For this review, take the finished solid that the model builds, in its own axes (mm). A direction names the side the tool comes from. Coordinates: 2 decimals unless noted, no trailing zeros. Write each loop counter-clockwise with the first axis right and the second up, starting at its lowest first coordinate (ties: lowest second). Pieces come first, ordered by that corner, then holes. Notation, with made-up numbers: (87, -39.5) - (114, -39.5) arc R38 cw to (114, -1.5) - close; hole circle Ø10 at (-25, 5). An arc over 180 degrees is marked (long way). Use one line per item in the form item = value. Start each with the question number.
1) For L1, parallel to Y at x = 0, z = -1; L2, parallel to Z at x = -1, y = -18.5; L3, parallel to Z at x = -15, y = 5.5, list the stretches that pass through material, from the lowest coordinate up. Write a range as from..to.
2) Tool access review of faces 5 (the flat face through (-17, 0, -52)), 6 (the cylindrical face through (-3.22, 24.54, -30.57)), 7 (the flat face through (0, -17, -5)): name each direction out of +Z, -Z, +X, -X, +Y, -Y from which nothing blocks a thin tool from reaching the whole face with its end or side.
3) We need section D-D (x = 17.5). Give the boundary of the cut face in (y, z), plus the area to 3 significant figures.
4) Insertion check: P1, Ø5, axis at x = 17.5, y = 0, coming from the -Z side; P2, Ø5, axis at y = 17.5, z = -47, coming from the -X side; P3, Ø4.5, axis at x = -17.5, y = 0, coming from the +Z side; P4, Ø10, axis at x = 5, y = 4, coming from the +Z side. Each pin has a flat end and moves straight along its axis. Give the tip position at first contact, or say it passes through.
5) We need section B-B (z = -58.5). Give the boundary of the cut face in (x, y), plus the area to 3 significant figures.
6) Mouldability with a two-part tool opening along X and no side actions: class faces 1 (the flat face through (0, 18, -5)), 2 (the cylindrical face through (1.172, 8.923, -65.451)), 3 (the flat face through (11, 0, -62)), 4 (the cylindrical face through (15.9, -1.2, -2.5)) as pulls with the +X half, pulls with the -X half, needs draft (parallel to the pull), parting line crosses it, or undercut.
7) We need section C-C (y = 17.5). Give the boundary of the cut face in (x, z), plus the area to 3 significant figures.
```python
from build123d import *

# Parameters (mm, degrees)
SKETCH1_R               = 24.75
BOSS_EXTRUDE1_DEPTH     = 62
SKETCH2_R               = 3
BOSS_EXTRUDE2_DEPTH     = 44
SKETCH3_R               = 1.1
CUT_EXTRUDE1_DEPTH      = 25.75
CUT_EXTRUDE1_DEPTH_BACK = 25.75
SKETCH4_R               = 9
BOSS_EXTRUDE3_DEPTH     = 7
SKETCH5_R               = 2
CUT_EXTRUDE2_DEPTH      = 10
SKETCH6_R               = 2
CUT_EXTRUDE3_DEPTH      = 5


with BuildPart() as part:
    # Sketch1 → Boss-Extrude1 (new body)
    with BuildSketch(Plane.XY):
        Circle(SKETCH1_R)
    extrude(amount=-BOSS_EXTRUDE1_DEPTH)

    # Sketch2 → Boss-Extrude2 (add)
    with BuildSketch(Plane.XY):
        Circle(SKETCH2_R)
    extrude(amount=BOSS_EXTRUDE2_DEPTH)

    # Sketch3 → Cut-Extrude1 (cut, two sides)
    with BuildSketch(Plane(origin=(0, 0, 0), x_dir=(0, 0, -1), z_dir=(1, 0, 0))) as cut_extrude1_sk:
        with Locations((-22, 0)):
            Circle(SKETCH3_R)
    extrude(amount=CUT_EXTRUDE1_DEPTH, mode=Mode.SUBTRACT)
    extrude(cut_extrude1_sk.sketch, amount=-CUT_EXTRUDE1_DEPTH_BACK, mode=Mode.SUBTRACT)

    # Sketch4 → Boss-Extrude3 (add)
    with BuildSketch(Plane(origin=(0, 0, -62), x_dir=(-1, 0, 0), z_dir=(0, 0, -1))):
        Circle(SKETCH4_R)
    extrude(amount=BOSS_EXTRUDE3_DEPTH)

    # Sketch5 → Cut-Extrude2 (cut)
    with BuildSketch(Plane(origin=(0, 0, -62), x_dir=(-1, 0, 0), z_dir=(0, 0, -1))):
        with Locations((-17.5, 0)):
            Circle(SKETCH5_R)
        with Locations((17.5, 0)):
            Circle(SKETCH5_R)
    extrude(amount=-CUT_EXTRUDE2_DEPTH, mode=Mode.SUBTRACT)

    # Sketch6 → Cut-Extrude3 (cut)
    with BuildSketch(Plane.XY):
        with Locations((0, 17.5)):
            Circle(SKETCH6_R)
        with Locations((17.5, 0)):
            Circle(SKETCH6_R)
        with Locations((0, -17.5)):
            Circle(SKETCH6_R)
        with Locations((-17.5, 0)):
            Circle(SKETCH6_R)
    extrude(amount=-CUT_EXTRUDE3_DEPTH, mode=Mode.SUBTRACT)


solid = part.part
```
Determined:
q1.L1 = -24.75..-19.5, -15.5..15.5, 19.5..24.75
q1.L2 = -62..-5
q1.L3 = -62..0
q2.face_5 = -Z
q2.face_6 = +Z, -Z
q2.face_7 = +Z
q3.outline = (-17.5, -62) - (-2, -62) - (-2, -52) - (2, -52) - (2, -62) - (17.5, -62) - (17.5, 0) - (2, 0) - (2, -5) - (-2, -5) - (-2, 0) - (-17.5, 0) - close
q3.area = 2,110 mm²
q4.P1 = -62
q4.P2 = -19.69
q4.P3 = 0
q4.P4 = 44
q5.outline = circle Ø49.5 at (0, 0); hole circle Ø4 at (-17.5, 0); hole circle Ø4 at (17.5, 0)
q5.area = 1,900 mm²
q6.face_1 = undercut
q6.face_2 = parting line crosses it
q6.face_3 = needs draft
q6.face_4 = undercut
q7.outline = (-17.5, -62) - (17.5, -62) - (17.5, 0) - (2, 0) - (2, -5) - (-2, -5) - (-2, 0) - (-17.5, 0) - close
q7.area = 2,150 mm²
